The model under review builds one solid part; all positions refer to its coordinate system, in mm. A direction names the side the tool comes from. Coordinates: 2 decimals unless noted, no trailing zeros. Order: outer loops, then holes, each group sorted by start corner. A loop starts at its lowest first (then second) coordinate and runs counter-clockwise, first axis right, second up. Notation, with made-up numbers: (35.25, 33) -> (91.25, 33) arc R25 ccw to (91.25, 51) -> close; hole circle Ø10 at (81.5, 63.25). An arc over 180 degrees is marked (long way). Use one line per item in the form item = value. Start each with the question number.
(1) Take a section at D-D (x = 56). State the section outline as (y, z) points.
(2) Take a section at B-B (y = 23). State the section outline as (x, z) points.
(3) For faces 1 (the flat face through (34.83, 7, 42)), 2 (the flat face through (17, 0, 29)), 3 (the cylindrical face through (37.84, -2.5, 9.95)), list the 3-axis set-ups (+Z, -Z, +X, -X, +Y, -Y) from which the entire face can be reached by the end or side of a thin tool; tool diameter is ignored.
(4) Take a section at A-A (z = 0). State the section outline as (x, y) points.
(5) Wall thickness on line 1 along Z through (x, y) = (24.5, 13); line 2 along Y through (x, z) = (50.23, -16.1); line 3 along Z through (x, y) = (35.5, 22): over which ranges is each line inside the solid? List them lowest first.
(6) Insertion check: pin 1 Ø4 at (y, z) = (-2, 0) entering from +X; pin 2 Ø8 at (x, y) = (45, -1) entering from +Z; pin 3 Ø1 at (x, y) = (37.5, -1.5) entering from -Z. Each pin has a flat end and moves straight along its axis. Give the tip position at first contact, or say it passes through.
(7) Take a section at C-C (y = 12.7). State the section outline as (x, z) points.
(8) Mouldability with a two-part tool opening along Z and no side actions: class faces 4 (the cylindrical face through (46.824, 13.773, 15.304)), 5 (the flat face through (17, 13, 40.38)), 6 (the flat face through (17, 10, 45.46)) as +Z half, -Z half, draft (parallel to the pull), parting line (faces both ways), or undercut.
```python
from build123d import *

# Parameters (mm, degrees)
BOSS_EXTRUDE1_DEPTH     = 34.83
SKETCH3_W               = 5.08
SKETCH3_H               = 30.48
BOSS_EXTRUDE2_DEPTH     = 25.4
F_1_4_CLEARANCE_HOLE1_D = 7.14248
CHAMFER1_SIZE           = 10
CHAMFER1_SIZE2          = 11.917535926
FILLET1_R               = 10
F_1_4_CLEARANCE_HOLE2_D = 7.14248


with BuildPart() as part:
    # Sketch2 → Boss-Extrude1 (new body)
    with BuildSketch(Plane(origin=(0, 0, 0), x_dir=(0, 0, -1), z_dir=(1, 0, 0))):
        Polygon((12.8, 0), (12.8, 25.4), (17.88, 25.4), (17.88, 0), (40.38, 0), (40.38, 25.4), (45.46, 25.4), (45.46, -5.08), (15.34, -5.08), (0, -5.08), (0, 0), align=None)
        Polygon((0, 0), (0, -5.08), (-15.34, -5.08), (-45.46, -5.08), (-45.46, 25.4), (-40.38, 25.4), (-40.38, 0), (-17.88, 0), (-17.88, 25.4), (-12.8, 25.4), (-12.8, 0), align=None)
    extrude(amount=BOSS_EXTRUDE1_DEPTH)

    # Sketch3 → Boss-Extrude2 (add)
    with BuildSketch(Plane(origin=(34.83, 0, 0), x_dir=(0, 0, -1), z_dir=(1, 0, 0))):
        with Locations((-15.34, 10.16)):
            Rectangle(SKETCH3_W, SKETCH3_H)
        with Locations((15.34, 10.16)):
            Rectangle(SKETCH3_W, SKETCH3_H)
    extrude(amount=BOSS_EXTRUDE2_DEPTH)

    # 1_4 Clearance Hole1 (through all)
    with Locations(Plane.XY.offset(17.88)):
        with Locations((50.23, 12.7)):
            Hole(F_1_4_CLEARANCE_HOLE1_D / 2)

    # Chamfer1
    chamfer1_edges = [part.edges().sort_by_distance(p)[0] for p in [
        (60.23, -5.08, 15.34),
        (60.23, -5.08, -15.34),
    ]]
    chamfer1_side = [part.faces().sort_by_distance(p)[0] for p in [
        (19.684206994, -5.08, 0),
    ]]
    chamfer(chamfer1_edges, length=CHAMFER1_SIZE, length2=CHAMFER1_SIZE2, reference=chamfer1_side[0])

    # Fillet1
    fillet1_edges = [part.edges().sort_by_distance(p)[0] for p in [
        (34.83, -2.54, 17.88),
        (34.83, -2.54, 12.8),
        (34.83, -2.54, -12.8),
        (34.83, -2.54, -17.88),
    ]]
    fillet(fillet1_edges, radius=FILLET1_R)

    # 1_4 Clearance Hole2 (through all)
    with Locations(Plane(origin=(0, -5.08, 0), x_dir=(-1, 0, 0), z_dir=(0, -1, 0))):
        with Locations((-17.415, 0)):
            Hole(F_1_4_CLEARANCE_HOLE2_D / 2)


solid = part.part
```
Findings:
q1.outline = (1.8, -17.88) -> (25.4, -17.88) -> (25.4, -12.8) -> (1.8, -12.8) -> close; (1.8, 12.8) -> (25.4, 12.8) -> (25.4, 17.88) -> (1.8, 17.88) -> close
q2.outline = (0, -45.46) -> (34.83, -45.46) -> (34.83, -40.38) -> (0, -40.38) -> close; (0, -17.88) -> (60.23, -17.88) -> (60.23, -12.8) -> (0, -12.8) -> close; (0, 12.8) -> (60.23, 12.8) -> (60.23, 17.88) -> (0, 17.88) -> close; (0, 40.38) -> (34.83, 40.38) -> (34.83, 45.46) -> (0, 45.46) -> close
q3.face_1 = +Z, +X, +Y, -Y
q3.face_2 = +X, -X, +Y
q3.face_3 = +X, +Y, -Y
q4.outline = (0, -5.08) -> (13.84, -5.08) -> (13.84, 0) -> (0, 0) -> close; (20.99, -5.08) -> (34.83, -5.08) -> (34.83, 0) -> (20.99, 0) -> close
q5.line_1 = -45.46 to -40.38, -17.88 to -12.8, 12.8 to 17.88, 40.38 to 45.46
q5.line_2 = -5.08 to 9.13, 16.27 to 25.4
q5.line_3 = -17.88 to -12.8, 12.8 to 17.88
q6.pin_1 = 34.83
q6.pin_2 = 18.64
q6.pin_3 = -21.66
q7.outline = (0, -45.46) -> (34.83, -45.46) -> (34.83, -40.38) -> (0, -40.38) -> close; (0, -17.88) -> (46.66, -17.88) -> (46.66, -12.8) -> (0, -12.8) -> close; (0, 12.8) -> (46.66, 12.8) -> (46.66, 17.88) -> (0, 17.88) -> close; (0, 40.38) -> (34.83, 40.38) -> (34.83, 45.46) -> (0, 45.46) -> close; (53.8, -17.88) -> (60.23, -17.88) -> (60.23, -12.8) -> (53.8, -12.8) -> close; (53.8, 12.8) -> (60.23, 12.8) -> (60.23, 17.88) -> (53.8, 17.88) -> close
q8.face_4 = draft
q8.face_5 = undercut
q8.face_6 = +Z half
